Can you work these out from the model? Positions are in its coordinate system, mm. Round coordinates to 2 decimals unless told otherwise and drop trailing zeros. Order: outer loops, then holes, each group sorted by start corner. A loop starts at its lowest first (then second) coordinate and runs counter-clockwise, first axis right, second up. Notation, with made-up numbers: M 81,-15 L 93,-15 A18 cw 93,3 Z; hole C 38,13.25 d2. An arc over 180 degrees is marked long. Answer as a JSON object with one key per item and string values. Group by question number.
```python
from build123d import *

# Parameters (mm, degrees)
ODEBRAT_VYSUNUT_M1_DEPTH      = 29.948229652
ODEBRAT_VYSUNUT_M1_DEPTH_BACK = 29.948229652
SKICA2_W                      = 9.5
SKICA2_H                      = 6.5


with BuildPart() as part:
    # Skica1 → Rotovat1 (revolve)
    with BuildSketch(Plane(origin=(0, 0, 0), x_dir=(0, 0, -1), z_dir=(1, 0, 0)), mode=Mode.PRIVATE) as rotovat1_sk:
        Polygon((0, 4), (0, 4.75), (-6.5, 4.75), (-6.5, 9), (-7.75, 9), (-8.75, 7.26), (-23.75, 7.26), (-24.75, 9), (-26, 9), (-26, 4), align=None)
    revolve(rotovat1_sk.sketch.rotate(Axis((0, 0, 0), (0, 0, 1)), 90), axis=Axis((0, 0, 0), (0, 0, 1)))

    # Skica2 → Odebrat vysunutím1 (cut, two sides: drawn at the far end of the back side and taken through both)
    with BuildSketch(Plane(origin=(0, 0, 0), x_dir=(1, 0, 0), z_dir=(0, 1, 0)).offset(-ODEBRAT_VYSUNUT_M1_DEPTH_BACK)):
        with Locations((0, -3.25)):
            Rectangle(SKICA2_W, SKICA2_H)
    extrude(amount=ODEBRAT_VYSUNUT_M1_DEPTH + ODEBRAT_VYSUNUT_M1_DEPTH_BACK, mode=Mode.SUBTRACT)


solid = part.part
```
1) I need wall thicknesses on line 1 along Y through (x, z) = (0, 17.5); line 2 along Y through (x, z) = (-0.5, 8); line 3 along Z through (x, y) = (-5, -5.75). Which ranges of each line are inside material? Lowest first, please.
2) If we section it at A-A on y = 0: Write out the boundary of the cut face in (x, z), plus the area to 3 significant figures.
3) If we section it at C-C on z = 15.5: Write out the boundary of the cut face in (x, y), plus the area to 3 significant figures.
4) For pin 1 (5 mm diameter, centred on y = 5, z = 17.5, fed in from +X); pin 2 (4 mm diameter, centred on y = 7, z = 15, fed in from -X); pin 3 (8 mm diameter, centred on y = 3, z = 11, fed in from +X), each with a flat end and sliding along its axis, tell me the tip position at first contact or that it passes through.
5) We'd pull the mould along Z, two halves only. Please class faces 1 (the face through (-2, 4, 26)), 2 (the face through (4, 2, 6.5)), 3 (the face through (-6.925, -2.181, 16.355)), 4 (the face through (6.633, -6.083, 7.134)): +Z half, -Z half, draft (parallel to the pull), parting line (faces both ways), or undercut.
Findings:
{
 "1": {"line 1": "y = -7.26 to -4, 4 to 7.26", "line 2": "y = -8.55 to -3.97, 3.97 to 8.55", "line 3": "z = 6.5 to 8.54, 23.96 to 26"},
 "2": {"outline": "M -9,6.5 L -4,6.5 L -4,26 L -9,26 L -9,24.75 L -7.26,23.75 L -7.26,8.75 L -9,7.75 Z; M 4,6.5 L 9,6.5 L 9,7.75 L 7.26,8.75 L 7.26,23.75 L 9,24.75 L 9,26 L 4,26 Z", "area": "139 mm^2"},
 "3": {"outline": "C 0,0 d14.52; hole C 0,0 d8", "area": "115 mm^2"},
 "4": {"pin 1": "stops at x = 6.82", "pin 2": "stops at x = -5.26", "pin 3": "stops at x = 8.98"},
 "5": {"face 1": "+Z half", "face 2": "-Z half", "face 3": "undercut", "face 4": "draft"}
}
